The model under review builds one solid part; all positions refer to its coordinate system, in mm. Coordinates: 2 decimals unless noted, no trailing zeros. Write each loop counter-clockwise with the first axis right and the second up, starting at its lowest first coordinate (ties: lowest second). Pieces come first, ordered by that corner, then holes.
1) Add section B-B, the plane z = 372. State the section outline as (x, y) points.
2) For line 1 (Y direction, x = 151, z = 419); line 2 (Y direction, x = 154, z = 284.5); line 3 (Y direction, x = 159.25, z = 225), list the stretches that pass through material, from the lowest coordinate up.
3) For P1, Ø7.5, axis at x = 153.5, y = 85, coming from the -Z side; P2, Ø4, axis at x = 151, y = 72.5, coming from the +Z side; P3, Ø4.5, axis at y = -10, z = 234.5, coming from the -X side, all flat-tipped, find the tip position at first contact; note any pin that passes through.
4) Add section D-D, the plane z = 199. State the section outline as (x, y) points, then the cut area to 3 significant figures.
5) Add section C-C, the plane y = 147.5. State the section outline as (x, z) points.
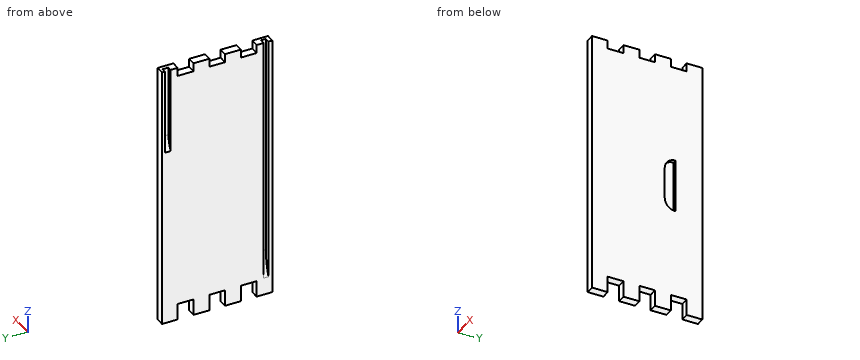
from build123d import *

# Parameters (mm, degrees)
ESQUISSE1_W             = 15.25
ESQUISSE1_H             = 205.5
BOSS_EXTRU_1_DEPTH      = 465.25
ESQUISSE2_W             = 30.5
ESQUISSE2_H             = 29.357142857
ESQUISSE2_H_2           = 29.357142858
BOSS_EXTRU_2_DEPTH      = 15.25
ENL_V_MAT_EXTRU_1_REACH = 17.25
ESQUISSE3_W             = 15.75
ESQUISSE3_H             = 29.357142857
ENL_V_MAT_EXTRU_2_DEPTH = 7
ESQUISSE5_W             = 8
ESQUISSE5_H             = 11
ENL_V_MAT_EXTRU_3_DEPTH = 160
ESQUISSE6_W             = 9.17735242
ESQUISSE6_H             = 9
ENL_V_MAT_EXTRU_4_DEPTH = 415.75
ESQUISSE7_R             = 127.5
ENL_V_MAT_EXTRU_5_DEPTH = 9
BOSS_EXTRU_3_REACH      = 18.25


with BuildPart() as part:
    # Esquisse1 → Boss.-Extru.1 (new body)
    with BuildSketch(Plane.XY):
        with Locations((155.460152838, 82.563864629)):
            Rectangle(ESQUISSE1_W, ESQUISSE1_H)
    extrude(amount=BOSS_EXTRU_1_DEPTH)

    # Esquisse2 → Boss.-Extru.2 (add)
    with BuildSketch(Plane(origin=(163.085152838, 0, 0), x_dir=(0, 0, -1), z_dir=(1, 0, 0))):
        with Locations((15.25, 170.635293201)):
            Rectangle(ESQUISSE2_W, ESQUISSE2_H)
        with Locations((15.25, 111.921007486)):
            Rectangle(ESQUISSE2_W, ESQUISSE2_H_2)
        with Locations((15.25, 53.206721771)):
            Rectangle(ESQUISSE2_W, ESQUISSE2_H)
        with Locations((15.25, -5.507563943)):
            Rectangle(ESQUISSE2_W, ESQUISSE2_H)
    extrude(amount=-BOSS_EXTRU_2_DEPTH)

    # Esquisse3 → Enlèv. mat.-Extru.1 (cut, up to next)
    with BuildSketch(Plane(origin=(163.085152838, 0, 0), x_dir=(0, 0, -1), z_dir=(1, 0, 0)), mode=Mode.PRIVATE) as enl_v_mat_extru_1_sk1:
        with Locations((-457.375, 141.278150344)):
            Rectangle(ESQUISSE3_W, ESQUISSE3_H)
    enl_v_mat_extru_1_tool1 = extrude(enl_v_mat_extru_1_sk1.sketch, amount=-ENL_V_MAT_EXTRU_1_REACH, mode=Mode.PRIVATE) & part.part
    add(enl_v_mat_extru_1_tool1.solids().sort_by_distance((163.085153, 141.27815, 457.375))[0], mode=Mode.SUBTRACT)
    # Esquisse3 → Enlèv. mat.-Extru.1 (cut, up to next)
    with BuildSketch(Plane(origin=(163.085152838, 0, 0), x_dir=(0, 0, -1), z_dir=(1, 0, 0)), mode=Mode.PRIVATE) as enl_v_mat_extru_1_sk2:
        with Locations((-457.375, 82.563864628)):
            Rectangle(ESQUISSE3_W, ESQUISSE3_H)
    enl_v_mat_extru_1_tool2 = extrude(enl_v_mat_extru_1_sk2.sketch, amount=-ENL_V_MAT_EXTRU_1_REACH, mode=Mode.PRIVATE) & part.part
    add(enl_v_mat_extru_1_tool2.solids().sort_by_distance((163.085153, 82.563865, 457.375))[0], mode=Mode.SUBTRACT)
    # Esquisse3 → Enlèv. mat.-Extru.1 (cut, up to next)
    with BuildSketch(Plane(origin=(163.085152838, 0, 0), x_dir=(0, 0, -1), z_dir=(1, 0, 0)), mode=Mode.PRIVATE) as enl_v_mat_extru_1_sk3:
        with Locations((-457.375, 23.849578915)):
            Rectangle(ESQUISSE3_W, ESQUISSE3_H)
    enl_v_mat_extru_1_tool3 = extrude(enl_v_mat_extru_1_sk3.sketch, amount=-ENL_V_MAT_EXTRU_1_REACH, mode=Mode.PRIVATE) & part.part
    add(enl_v_mat_extru_1_tool3.solids().sort_by_distance((163.085153, 23.849579, 457.375))[0], mode=Mode.SUBTRACT)

    # Esquisse4 → Enlèv. mat.-Extru.2 (cut)
    with BuildSketch(Plane(origin=(163.085152838, 0, 0), x_dir=(0, 0, -1), z_dir=(1, 0, 0))):
        with BuildLine():
            Line((-267.375, 135.313864629), (-167.375, 135.313864629))
            ThreePointArc((-167.375, 135.313864629), (-173.232864376, 121.171729005), (-187.375, 115.313864629))
            Line((-187.375, 115.313864629), (-247.375, 115.313864629))
            ThreePointArc((-247.375, 115.313864629), (-261.517135624, 121.171729005), (-267.375, 135.313864629))
        make_face()
    extrude(amount=-ENL_V_MAT_EXTRU_2_DEPTH, mode=Mode.SUBTRACT)

    # Esquisse5 → Enlèv. mat.-Extru.3 (cut)
    with BuildSketch(Plane.XY.offset(465.25)):
        with Locations((151.835152838, 174.563864629)):
            Rectangle(ESQUISSE5_W, ESQUISSE5_H)
    extrude(amount=-ENL_V_MAT_EXTRU_3_DEPTH, mode=Mode.SUBTRACT)

    # Esquisse6 → Enlèv. mat.-Extru.4 (cut)
    with BuildSketch(Plane.XY.offset(465.25)):
        with Locations((152.423829048, -8.436135371)):
            Rectangle(ESQUISSE6_W, ESQUISSE6_H)
    extrude(amount=-ENL_V_MAT_EXTRU_4_DEPTH, mode=Mode.SUBTRACT)

    # Esquisse7 → Enlèv. mat.-Extru.5 (cut)
    with BuildSketch(Plane.XZ.offset(3.936135371)):
        with Locations((29.512505258, 49.5)):
            Circle(ESQUISSE7_R)
    extrude(amount=ENL_V_MAT_EXTRU_5_DEPTH, mode=Mode.SUBTRACT)

    # Esquisse8 → Boss.-Extru.3 (add, up to next)
    with BuildSketch(Plane(origin=(0, 169.063864629, 0), x_dir=(1, 0, 0), z_dir=(0, 1, 0)), mode=Mode.PRIVATE) as boss_extru_3_sk1:
        with BuildLine():
            Line((147.835152838, -305.25), (155.835152838, -305.25))
            Line((155.835152838, -305.25), (155.835152838, -332.922407507))
            ThreePointArc((155.835152838, -332.922407507), (153.795024483, -318.519611448), (147.835152838, -305.25))
        make_face()
    boss_extru_3_tool1 = extrude(boss_extru_3_sk1.sketch, amount=BOSS_EXTRU_3_REACH, mode=Mode.PRIVATE) - part.part
    add(boss_extru_3_tool1.solids().sort_by_distance((153.470601, 169.063865, 312.056849))[0])


solid = part.part
Geometry results:
1. outline: (147.84, -20.19) - (163.09, -20.19) - (163.09, 185.31) - (147.84, 185.31) - (147.84, 180.06) - (155.84, 180.06) - (155.84, 169.06) - (147.84, 169.06) - (147.84, -3.94) - (157.01, -3.94) - (157.01, -12.94) - (147.84, -12.94) - close
2. line 1: y = -20.19 to -12.94, -3.94 to 169.06, 180.06 to 185.31
2. line 2: y = -20.19 to -12.94, -3.94 to 185.31
2. line 3: y = -20.19 to 115.31, 135.31 to 185.31
3. P1: stops at z = 0
3. P2: stops at z = 449.5
3. P3: stops at x = 157.01
4. outline: (147.84, -20.19) - (163.09, -20.19) - (163.09, 115.31) - (156.09, 115.31) - (156.09, 135.31) - (163.09, 135.31) - (163.09, 185.31) - (147.84, 185.31) - (147.84, -3.94) - (157.01, -3.94) - (157.01, -12.94) - (147.84, -12.94) - close
4. area: 2,910 mm2
5. outline: (147.84, 0) - (163.09, 0) - (163.09, 449.5) - (147.84, 449.5) - close
